from build123d import *

# Parameters (mm, degrees)
F0_W     = 100
F0_H     = 101.4652305061
F1_DEPTH = 100
F2_R     = 25
F3_DEPTH = 50
F4_R     = 25
F5_DEPTH = 50
F7_DEPTH = 25.4
F8_R     = 25
F9_DEPTH = 25.4


# Not quite as in the source:
# - the program builds the solid bodies; features that only make, move or delete a surface that nothing else refers to are left out


with BuildPart() as f1:
    # F0 (on Top) → F1 (new body)
    with BuildSketch(Plane.XY):
        Rectangle(F0_W, F0_H)
    extrude(amount=F1_DEPTH)

    # F2 (on face) → F3 (join)
    with BuildSketch(Plane.XY.offset(100)):
        Circle(F2_R)
    extrude(amount=F3_DEPTH)

    # F4 (on Top) → F5 (join)
    with BuildSketch(Plane.XY):
        Circle(F4_R)
    extrude(amount=F5_DEPTH)

    # F4 (on Top) → F7 (join)
    with BuildSketch(Plane.XY):
        Circle(F4_R)
    extrude(amount=F7_DEPTH)

    # F8 (on face) → F9 (cut)
    with BuildSketch(Plane.YZ.offset(50)):
        with Locations((0, 47.2276035258)):
            Circle(F8_R)
    extrude(amount=-F9_DEPTH, mode=Mode.SUBTRACT)


solid = f1.part
The listing builds one solid part. Answer for the finished solid, in the listing's coordinates (mm). A direction names the side the tool comes from. Round coordinates to 2 decimals unless told otherwise and drop trailing zeros. Order: outer loops, then holes, each group sorted by start corner. A loop starts at its lowest first (then second) coordinate and runs counter-clockwise, first axis right, second up. Notation, with made-up numbers: (28.5, 1) -> (54.5, 1) arc R21 cw to (54.5, 19) -> close; hole circle Ø4 at (-38.5, -36.75). An arc over 180 degrees is marked (long way). One line per item, written item: value.
Item 1: Find section D-D, the plane y = -35.5. Give the vertices of the cut face in (x, z), then the cut area to 3 significant figures.
Taken from the geometry:
outline: (-50, 0) -> (50, 0) -> (50, 100) -> (-50, 100) -> close
area: 10,000 mm2
Item 2: Given P1, Ø2, axis at x = -18, y = 33.5, coming from the +Z side; P2, Ø4, axis at y = 5.5, z = 128, coming from the -X side; P3, Ø8, axis at y = -14, z = 32.5, coming from the +X side, each flat-ended and moving along its own axis, determine where each tip first touches the part or whether it passes through.
Taken from the geometry:
P1: stops at z = 100
P2: stops at x = -24.75
P3: stops at x = 24.6
Item 3: Find section C-C, the plane z = 27. Give the vertices of the cut face in (x, y).
Taken from the geometry:
outline: (-50, -50.73) -> (50, -50.73) -> (50, -14.69) -> (24.6, -14.69) -> (24.6, 14.69) -> (50, 14.69) -> (50, 50.73) -> (-50, 50.73) -> close
Item 4: Find section A-A, the plane x = 0. Give the vertices of the cut face in (y, z).
Taken from the geometry:
outline: (-50.73, 0) -> (50.73, 0) -> (50.73, 100) -> (25, 100) -> (25, 150) -> (-25, 150) -> (-25, 100) -> (-50.73, 100) -> close
Item 5: Find section B-B, the plane y = 0. Give the vertices of the cut face in (x, z), then the cut area to 3 significant figures.
Taken from the geometry:
outline: (-50, 0) -> (50, 0) -> (50, 22.23) -> (24.6, 22.23) -> (24.6, 72.23) -> (50, 72.23) -> (50, 100) -> (25, 100) -> (25, 150) -> (-25, 150) -> (-25, 100) -> (-50, 100) -> close
area: 11,200 mm2
Item 6: Straight lines are drawn through the part: L1, parallel to Z at x = 33, y = 0; L2, parallel to X at y = -11.5, z = 55; L3, parallel to Z at x = -35.5, y = 2. For each, find the intervals that lie inside material, in ascending order.
Taken from the geometry:
L1: z = 0 to 22.23, 72.23 to 100
L2: x = -50 to 24.6
L3: z = 0 to 100
Item 7: For a pull along Y with two mould halves and no side action, classify faces 4 (the flat face through (24.6, 0, 48)), 5 (the flat face through (-1, 50.733, 49)), 6 (the flat face through (-1, -50.733, 49)) as released by +Y, released by -Y, zero draft, split by the parting line, or undercut.
Taken from the geometry:
face 4: undercut
face 5: released by +Y
face 6: released by -Y
Item 8: For faces 1 (the flat face through (-23, 12, 100)), 2 (the flat face through (50, -12, 72)), 3 (the cylindrical face through (37.478, -3.255, 72.015)), determine the directions among +Z, -Z, +X, -X, +Y, -Y from which every point of the face is accessible in a straight line to the end or side of a thin tool.
Taken from the geometry:
face 1: +Z
face 2: +Z, -Z, +X, +Y, -Y
face 3: +X
